Design review of the part shown in the three views and the two pictorial views. Dimensions are in mm from the part's minimum x, y and z. Round coordinates to 2 decimals unless told otherwise and drop trailing zeros. Order: outer loops, then holes, each group sorted by start corner. A loop starts at its lowest first (then second) coordinate and runs counter-clockwise, first axis right, second up.
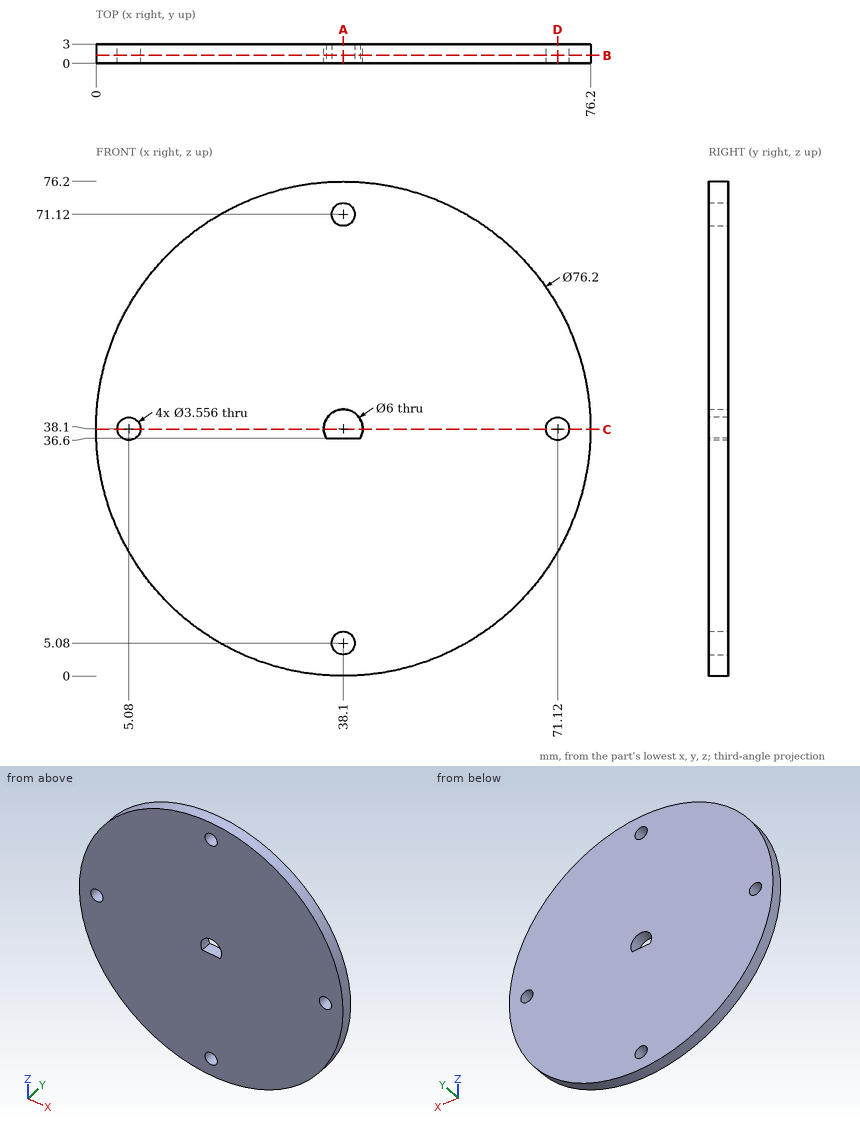
(1) Wall thickness on L1, parallel to X at y = 1.85, z = 38.1; L2, parallel to X at y = 1.35, z = 5.08; L3, parallel to X at y = 1.4, z = 49.5: over which ranges is each line inside the solid? List them lowest first.
(2) Add section A-A on x = 38.1. Give the boundary of the cut face in (y, z), plus the area to 3 significant figures.
(3) Add section B-B on y = 1.25. Give the boundary of the cut face in (x, z).
(4) Add section C-C on z = 38. Give the boundary of the cut face in (x, y), plus the area to 3 significant figures.
(5) Clearance check with a flat-ended pin moving along its axis: P1, Ø3, axis at x = 5.08, z = 38.1, coming from the +Y side. State where the tip first meets the part, or that it passes through.
(6) Add section D-D on x = 71.12. Give the boundary of the cut face in (y, z), plus the area to 3 significant figures.
Here are the results:
1. L1: x = 0 to 3.3, 6.86 to 35.1, 41.1 to 69.34, 72.9 to 76.2
1. L2: x = 19.09 to 36.32, 39.88 to 57.11
1. L3: x = 1.75 to 74.45
2. outline: (0, 0) - (3, 0) - (3, 3.3) - (0, 3.3) - close; (0, 6.86) - (3, 6.86) - (3, 36.6) - (0, 36.6) - close; (0, 41.1) - (3, 41.1) - (3, 69.34) - (0, 69.34) - close; (0, 72.9) - (3, 72.9) - (3, 76.2) - (0, 76.2) - close
2. area: 194 mm2
3. outline: circle Ø76.2 at (38.1, 38.1); hole circle Ø3.56 at (5.08, 38.1); hole (35.5, 36.6) - (40.7, 36.6) arc R3 ccw (long way) to start; hole circle Ø3.56 at (38.1, 5.08); hole circle Ø3.56 at (38.1, 71.12); hole circle Ø3.56 at (71.12, 38.1)
4. outline: (0, 0) - (3.3, 0) - (3.3, 3) - (0, 3) - close; (6.86, 0) - (35.1, 0) - (35.1, 3) - (6.86, 3) - close; (41.1, 0) - (69.34, 0) - (69.34, 3) - (41.1, 3) - close; (72.9, 0) - (76.2, 0) - (76.2, 3) - (72.9, 3) - close
4. area: 189 mm2
5. P1: passes through
6. outline: (0, 19.09) - (3, 19.09) - (3, 36.32) - (0, 36.32) - close; (0, 39.88) - (3, 39.88) - (3, 57.11) - (0, 57.11) - close
6. area: 103 mm2
